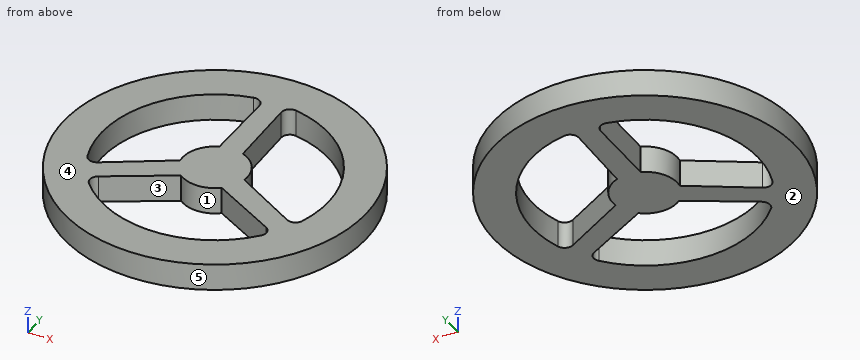
```python
from build123d import *

# Parameters (mm, degrees)
SKETCH_R     = 17.78
PAD_DEPTH    = 3.175
FILLET_R     = 1.016
SKETCH001_R  = 3.81
PAD001_DEPTH = 3.175


with BuildPart() as part:
    # Sketch → Pad (new body)
    with BuildSketch(Plane.XY):
        Circle(SKETCH_R)
        with BuildLine():
            Line((-1.27, 13.274386), (-1.394671, 1.88415))
            ThreePointArc((-2.329057, 0.265745), (-1.649778, 0.9525), (-1.394671, 1.88415))
            Line((-2.329057, 0.265745), (-12.130956, -5.537341))
            ThreePointArc((-1.27, 13.274386), (-11.548449, 6.6675), (-12.130956, -5.537341))
        make_face(mode=Mode.SUBTRACT)
        with BuildLine():
            Line((1.27, 13.274386), (1.394671, 1.88415))
            ThreePointArc((1.394671, 1.88415), (1.649778, 0.9525), (2.329057, 0.265745))
            Line((2.329057, 0.265745), (12.130956, -5.537341))
            ThreePointArc((12.130956, -5.537341), (11.548449, 6.6675), (1.27, 13.274386))
        make_face(mode=Mode.SUBTRACT)
        with BuildLine():
            Line((-0.934387, -2.149896), (-10.860956, -7.737045))
            ThreePointArc((-10.860956, -7.737045), (0, -13.335), (10.860956, -7.737045))
            Line((0.934387, -2.149896), (10.860956, -7.737045))
            ThreePointArc((0.934387, -2.149896), (0, -1.905), (-0.934387, -2.149896))
        make_face(mode=Mode.SUBTRACT)
    extrude(amount=PAD_DEPTH)

    # Fillet
    fillet_edges = [part.edges().sort_by_distance(p)[0] for p in [
        (-12.130956, -5.537341, 1.5875),
        (-1.27, 13.274386, 1.5875),
        (1.27, 13.274386, 1.5875),
        (-10.860956, -7.737045, 1.5875),
        (10.860956, -7.737045, 1.5875),
        (12.130956, -5.537341, 1.5875),
    ]]
    fillet(fillet_edges, radius=FILLET_R)

    # Sketch001 (on Face5 of Fillet) → Pad001 (join)
    with BuildSketch(Plane.XY.offset(3.175)):
        Circle(SKETCH001_R)
    extrude(amount=-PAD001_DEPTH)


solid = part.part
```
Part model, mm, in its own coordinate system. Face numbers are marked on the shaded views. A direction names the side the tool comes from. Round coordinates to 2 decimals unless told otherwise and drop trailing zeros. Loops run counter-clockwise (first coordinate to the right, second up) from the corner with the lowest first, then second, coordinate; pieces in that order, holes last.
Item 1: Drill centre lines: line 1 (X direction, y = 3.5, z = 1.9); line 2 (Y direction, x = 5.5, z = 1.95); line 3 (Y direction, x = -9.5, z = 0.85). Where is each one in solid material? Low to high.
Item 2: Cut at C-C, the plane z = 2.05. Give the cut face in (x, y) (3 decimals), then the cut area to 3 significant figures.
Item 3: Cut at B-B, the plane y = 0. Give the cut face in (x, z) (3 decimals).
Item 4: Mould opens along X. For the marked faces 3, 4 and 5 say: +X half, -X half, draft (parallel to the pull), parting line (faces both ways), or undercut.
Item 5: Drop a flat-ended pin along its axis: P1, Ø1.5, axis at y = -4.5, z = 1, coming from the +X side. Give the stop position or say it passes through.
Item 6: 3-axis set-ups, long thin cutter, end or side, ignore diameter. For the marked faces 1 and 2: which of +Z, -Z, +X, -X, +Y, -Y reach the whole face in a straight line?
Item 7: Cut at D-D, the plane y = -11. Give the cut face in (x, z) (3 decimals), then the cut area to 3 significant figures.
Item 8: Cut at A-A, the plane x = 0. Give the cut face in (y, z) (3 decimals).
A:
1. line 1: x = -17.43 to -12.87, -1.51 to 1.51, 12.87 to 17.43
1. line 2: y = -16.91 to -12.15, -4.72 to -1.61, 12.15 to 16.91
1. line 3: y = -15.03 to -9.36, -6.97 to -3.98, 9.36 to 15.03
2. outline: circle Ø35.56 at (0, 0); hole (-12.59, -4.395) arc R1.016 ccw to (-11.113, -4.935) - (-3.765, -0.584) arc R3.81 cw to (-1.376, 3.553) - (-1.283, 12.091) arc R1.016 ccw to (-2.488, 13.101) arc R13.335 ccw to start; hole (-10.101, -8.705) arc R13.335 ccw to (10.101, -8.705) arc R1.016 ccw to (9.83, -7.157) - (2.389, -2.968) arc R3.81 cw to (-2.389, -2.968) - (-9.83, -7.157) arc R1.016 ccw to start; hole (1.283, 12.091) - (1.376, 3.553) arc R3.81 cw to (3.765, -0.584) - (11.113, -4.935) arc R1.016 ccw to (12.59, -4.395) arc R13.335 ccw to (2.488, 13.101) arc R1.016 ccw to start
2. area: 558 mm2
3. outline: (-17.78, 0) - (-13.335, 0) - (-13.335, 3.175) - (-17.78, 3.175) - close; (-3.81, 0) - (3.81, 0) - (3.81, 3.175) - (-3.81, 3.175) - close; (13.335, 0) - (17.78, 0) - (17.78, 3.175) - (13.335, 3.175) - close
4. face 3: undercut
4. face 4: draft
4. face 5: parting line
5. P1: stops at x = 17.38
6. face 1: +Z, -Z
6. face 2: -Z, +X, -X, +Y, -Y
7. outline: (-13.969, 0) - (-7.538, 0) - (-7.538, 3.175) - (-13.969, 3.175) - close; (7.538, 0) - (13.969, 0) - (13.969, 3.175) - (7.538, 3.175) - close
7. area: 40.8 mm2
8. outline: (-17.78, 0) - (-13.335, 0) - (-13.335, 3.175) - (-17.78, 3.175) - close; (-3.81, 0) - (17.78, 0) - (17.78, 3.175) - (-3.81, 3.175) - close
